The model under review builds one solid part; all positions refer to its coordinate system, in mm. A direction names the side the tool comes from. Round coordinates to 2 decimals unless told otherwise and drop trailing zeros. Loops run counter-clockwise (first coordinate to the right, second up) from the corner with the lowest first, then second, coordinate; pieces in that order, holes last. Notation, with made-up numbers: (88, 34.5) -> (118, 34.5) arc R17 cw to (118, 41.5) -> close; hole circle Ø4 at (-14.75, -19.5). An arc over 180 degrees is marked (long way). Use a Markdown table: item, result. Add a question column.
1) For faces 1 (the cylindrical face through (0.66, 2.465, 15.425)), 2 (the flat face through (1.9, 0, 11.5)), list the 3-axis set-ups (+Z, -Z, +X, -X, +Y, -Y) from which the entire face can be reached by the end or side of a thin tool; tool diameter is ignored.
2) Consider section C-C on z = 14. Give the boundary of the cut face in (x, y).
3) Consider section B-B on x = 0. Give the boundary of the cut face in (y, z).
4) Insertion check: pin 1 (8 mm diameter, centred on x = 2, y = 18.5, fed in from -Z); pin 2 (4 mm diameter, centred on y = 4, z = -9.5, fed in from +X); pin 3 (12 mm diameter, centred on y = 16, z = 11, fed in from -X); pin 4 (3 mm diameter, centred on y = 8, z = -3, fed in from -X). Each pin has a flat end and moves straight along its axis. Give the tip position at first contact, or say it passes through.
5) Consider section A-A on z = 0. Give the boundary of the cut face in (x, y).
6) Consider section D-D on y = 25.75. Give the boundary of the cut face in (x, z), plus the area to 3 significant figures.
7) Wall thickness on probe 1 along Z at (x, y) = (-1, 22.25); probe 2 along Y at (x, z) = (-5.5, -12.5); probe 3 along X at (y, z) = (10.75, 1): over which ranges is each line inside the solid? List them lowest first.
8) Mouldability with a two-part tool opening along X and no side actions: class faces 3 (the flat face through (-8, 30, 8)), 4 (the cylindrical face through (-10.648, 14.79, -13.887)), 5 (the conical face through (9.735, 14.79, 3.066)) as released by +X, released by -X, zero draft, split by the parting line, or undercut.
from build123d import *

# Parameters (mm, degrees)
SKETCH2_R           = 17.5
BOSS_EXTRUDE2_DEPTH = 30
SKETCH3_R           = 11.5
CUT_EXTRUDE1_DEPTH  = 30
CUT_EXTRUDE1_DRAFT  = -5
SKETCH4_R           = 15
SKETCH4_R_2         = 12.5
CUT_EXTRUDE2_DEPTH  = 5


with BuildPart() as part:
    # Sketch2 → Boss-Extrude2 (new body)
    with BuildSketch(Plane(origin=(0, 0, 0), x_dir=(1, 0, 0), z_dir=(0, 1, 0))):
        with Locations(Location((0, 0, 0), (0, 0, 270))):
            Circle(SKETCH2_R)
    extrude(amount=BOSS_EXTRUDE2_DEPTH)


with BuildPart() as cut_extrude1_tool:
    # Sketch3 → Cut-Extrude1 (with draft: the straight prism first)
    with BuildSketch(Plane.XZ):
        Circle(SKETCH3_R)
    extrude(amount=-CUT_EXTRUDE1_DEPTH)
    # Cut-Extrude1: the draft: its side faces are tilted about the plane it starts from
    cut_extrude1_sides = [cut_extrude1_tool.faces().sort_by_distance(p)[0] for p in [
        (-11.5, 15, 0),
    ]]
    draft(cut_extrude1_sides, Plane.XZ, CUT_EXTRUDE1_DRAFT)


with BuildPart() as part_1:
    add(part.part)

    # Cut-Extrude1: cut by cut_extrude1_tool
    add(cut_extrude1_tool.part, mode=Mode.SUBTRACT)

    # Sketch4 → Cut-Extrude2 (cut)
    with BuildSketch(Plane.XZ):
        with Locations(Location((0, 0.439504446, 0), (0, 0, 270))):
            Circle(SKETCH4_R)
        with Locations(Location((0, 0.439504446, 0), (0, 0, 270))):
            Circle(SKETCH4_R_2, mode=Mode.SUBTRACT)
    extrude(amount=-CUT_EXTRUDE2_DEPTH, mode=Mode.SUBTRACT)


solid = part_1.part
Result set:
| question | item | result |
|---|---|---|
| 1 | face 1 | -Y |
| 1 | face 2 | +Z, -Z, +X, -X, -Y |
| 2 | outline | (-10.5, 0) -> (-6.41, 0) -> (-6.41, 5) -> (6.41, 5) -> (6.41, 0) -> (10.5, 0) -> (10.5, 30) -> (-10.5, 30) -> close |
| 3 | outline | (0, -17.5) -> (30, -17.5) -> (30, -8.88) -> (0, -11.5) -> (0, -12.06) -> (5, -12.06) -> (5, -14.56) -> (0, -14.56) -> close; (0, 11.5) -> (30, 8.88) -> (30, 17.5) -> (0, 17.5) -> (0, 15.44) -> (5, 15.44) -> (5, 12.94) -> (0, 12.94) -> close |
| 4 | pin 1 | z = -17.5 |
| 4 | pin 2 | x = 15.81 |
| 4 | pin 3 | x = -16.77 |
| 4 | pin 4 | x = -17.44 |
| 5 | outline | (-17.5, 0) -> (-14.99, 0) -> (-14.99, 5) -> (-12.49, 5) -> (-12.49, 0) -> (-11.5, 0) -> (-8.88, 30) -> (-17.5, 30) -> close; (8.88, 30) -> (11.5, 0) -> (12.49, 0) -> (12.49, 5) -> (14.99, 5) -> (14.99, 0) -> (17.5, 0) -> (17.5, 30) -> close |
| 6 | outline | circle Ø35 at (0, 0); hole circle Ø18.49 at (0, 0) |
| 6 | area | 693 mm2 |
| 7 | probe 1 | -17.47 to -9.5, 9.5 to 17.47 |
| 7 | probe 2 | 5 to 30 |
| 7 | probe 3 | -17.47 to -10.51, 10.51 to 17.47 |
| 8 | face 3 | zero draft |
| 8 | face 4 | split by the parting line |
| 8 | face 5 | undercut |
